Verification items for the finished model (mm, model axes). A direction names the side the tool comes from. Round coordinates to 2 decimals unless told otherwise and drop trailing zeros. Write each loop counter-clockwise with the first axis right and the second up, starting at its lowest first coordinate (ties: lowest second). Pieces come first, ordered by that corner, then holes.
from build123d import *

# Parameters (mm, degrees)
BOSS_EXTRUDE2_DEPTH   = 609.6
CUT_EXTRUDE1_DEPTH    = 1118.235
CUT_EXTRUDE2_REACH    = 612.426
SKETCH6_W             = 31.75
SKETCH6_H             = 31.75
F_6_CLEARANCE_HOLE1_D = 4.3053


with BuildPart() as part:
    # Sketch3 → Boss-Extrude2 (new, symmetric)
    with BuildSketch(Plane.XY):
        Polygon((-19.05, 12.7), (-19.05, -12.7), (19.05, -12.7), (19.05, 12.7), (15.875, 12.7), (15.875, -9.525), (-15.875, -9.525), (-15.875, 12.7), align=None)
    extrude(amount=BOSS_EXTRUDE2_DEPTH, both=True)

    # Sketch5 → Cut-Extrude1 (cut)
    with BuildSketch(Plane.XY.offset(609.6)):
        Polygon((-19.05, 12.7), (-15.875, 12.7), (-15.875, -9.525), (15.875, -9.525), (15.875, 12.7), (19.05, 12.7), (19.05, -12.7), (-19.05, -12.7), align=None)
    extrude(amount=-CUT_EXTRUDE1_DEPTH, mode=Mode.SUBTRACT)

    # Sketch6 → Cut-Extrude2 (cut, up to next)
    with BuildSketch(Plane.XZ.offset(12.7), mode=Mode.PRIVATE) as cut_extrude2_sk1:
        with Locations((0, -593.725)):
            Rectangle(SKETCH6_W, SKETCH6_H)
    cut_extrude2_tool1 = extrude(cut_extrude2_sk1.sketch, amount=-CUT_EXTRUDE2_REACH, mode=Mode.PRIVATE) & part.part
    add(cut_extrude2_tool1.solids().sort_by_distance((0, -12.7, -593.725))[0], mode=Mode.SUBTRACT)

    # #6 Clearance Hole1 (through all)
    with Locations(Plane(origin=(19.05, 0, 0), x_dir=(0, 0, -1), z_dir=(1, 0, 0))):
        with Locations((521.335, 0)):
            Hole(F_6_CLEARANCE_HOLE1_D / 2)


solid = part.part
Q1. Release check for a two-part mould opening along X. For faces 3 (the flat face through (15.875, 0, -558)), 4 (the flat face through (19.05, 0, -558)), 5 (the flat face through (17, 12.7, -558)), 6 (the flat face through (0, -11, -577.85)) record: released by +X, released by -X, zero draft, split by the parting line, or undercut.
Recorded:
face 3: undercut
face 4: released by +X
face 5: zero draft
face 6: undercut
Q2. Depth check by flat-ended pin: P1, Ø16, axis at x = 4.5, z = -549.5, coming from the +Y side (3 decimals); P2, Ø3.5, axis at x = -6, y = -11.5, coming from the -Z side. Enter the tip coordinate at first touch or a pass-through.
Recorded:
P1: stops at y = -9.525
P2: stops at z = -577.85
Q3. Material ranges on line 1 along X through (y, z) = (11.25, -568) (3 decimals); line 2 along Y through (x, z) = (-8, -575) (3 decimals), recorded low to high.
Recorded:
line 1: x = -19.05 to -15.875, 15.875 to 19.05
line 2: y = -12.7 to -9.525
Q4. Sectioned sample at D-D (z = -564.5). Enter the section's corners in (x, y) (3 decimals).
Recorded:
outline: (-19.05, -12.7) - (19.05, -12.7) - (19.05, 12.7) - (15.875, 12.7) - (15.875, -9.525) - (-15.875, -9.525) - (-15.875, 12.7) - (-19.05, 12.7) - close
Q5. Sectioned sample at A-A (z = -589.5). Enter the section's corners in (x, y) (3 decimals), plus the area to 3 significant figures.
Recorded:
outline: (-19.05, -12.7) - (-15.875, -12.7) - (-15.875, 12.7) - (-19.05, 12.7) - close; (15.875, -12.7) - (19.05, -12.7) - (19.05, 12.7) - (15.875, 12.7) - close
area: 161 mm2
Q6. Sectioned sample at B-B (y = -5). Enter the section's corners in (x, z) (3 decimals).
Recorded:
outline: (-19.05, -609.6) - (-15.875, -609.6) - (-15.875, -508.635) - (-19.05, -508.635) - close; (15.875, -609.6) - (19.05, -609.6) - (19.05, -508.635) - (15.875, -508.635) - close
Q7. Sectioned sample at C-C (y = 0). Enter the section's corners in (x, z) (3 decimals), plus the area to 3 significant figures.
Recorded:
outline: (-19.05, -609.6) - (-15.875, -609.6) - (-15.875, -523.488) - (-19.05, -523.488) - close; (-19.05, -519.182) - (-15.875, -519.182) - (-15.875, -508.635) - (-19.05, -508.635) - close; (15.875, -609.6) - (19.05, -609.6) - (19.05, -523.488) - (15.875, -523.488) - close; (15.875, -519.182) - (19.05, -519.182) - (19.05, -508.635) - (15.875, -508.635) - close
area: 614 mm2
Q8. Tool access check on faces 1 (the flat face through (-17, 0, -609.6)), 2 (the flat face through (0, -9.525, -543)). Record the directions out of +Z, -Z, +X, -X, +Y, -Y that give a thin tool (end or side, any length) a straight path to the whole face; none if there is none.
Recorded:
face 1: -Z, +X, -X, +Y, -Y
face 2: +Z, -Z, +Y
